Verification items for the finished model (mm, model axes). Coordinates: 2 decimals unless noted, no trailing zeros. Order: outer loops, then holes, each group sorted by start corner. A loop starts at its lowest first (then second) coordinate and runs counter-clockwise, first axis right, second up. Notation, with made-up numbers: (45, 36.25) -> (73, 36.25) arc R23 cw to (73, 75.25) -> close; hole circle Ø6 at (59.25, 60). An arc over 180 degrees is marked (long way). Answer as CSV lines item,"result".
```python
from build123d import *

# Parameters (mm, degrees)
SKETCH1_R           = 4
BOSS_EXTRUDE1_DEPTH = 6


with BuildPart() as part:
    # Sketch1 → Boss-Extrude1 (new body)
    with BuildSketch(Plane.XY):
        with BuildLine():
            Line((-80, 0), (-17.5, 0))
            ThreePointArc((-17.5, 0), (0, 17.5), (17.5, 0))
            Line((17.5, 0), (80, 0))
            ThreePointArc((80, 0), (0, 80), (-80, 0))
        make_face()
        with Locations((24.874423104, 60.052169613)):
            Circle(SKETCH1_R, mode=Mode.SUBTRACT)
        with Locations((60.052169613, 24.874423104)):
            Circle(SKETCH1_R, mode=Mode.SUBTRACT)
        with Locations((-60.052169613, 24.874423104)):
            Circle(SKETCH1_R, mode=Mode.SUBTRACT)
        with Locations(Location((-24.874423104, 60.052169613, 0), (0, 0, 180))):
            Circle(SKETCH1_R, mode=Mode.SUBTRACT)
    extrude(amount=BOSS_EXTRUDE1_DEPTH)


solid = part.part
```
Item 1: Section check B-B, the plane z = 3.6. Record the boundary of the cut face in (x, y).
Answer list:
outline,"(-80, 0) -> (-17.5, 0) arc R17.5 cw to (17.5, 0) -> (80, 0) arc R80 ccw to start; hole circle Ø8 at (-60.05, 24.87); hole circle Ø8 at (-24.87, 60.05); hole circle Ø8 at (24.87, 60.05); hole circle Ø8 at (60.05, 24.87)"
Item 2: Section check C-C, the plane x = 0. Record the boundary of the cut face in (y, z), plus the area to 3 significant figures.
Answer list:
outline,"(17.5, 0) -> (80, 0) -> (80, 6) -> (17.5, 6) -> close"
area,"375 mm2"
Item 3: Thickness scan on line 1 (X direction, y = 59.5, z = 5.7); line 2 (X direction, y = 5, z = 4.45); line 3 (X direction, y = 27, z = 1.6). Record the ranges inside material, lowest first.
Answer list:
line 1,"-53.48 to -28.84, -20.91 to 20.91, 28.84 to 53.48"
line 2,"-79.84 to -16.77, 16.77 to 79.84"
line 3,"-75.31 to -63.44, -56.66 to 56.66, 63.44 to 75.31"
Item 4: Depth check by flat-ended pin: pin 1 Ø4 at (x, y) = (28.5, 24) entering from -Z; pin 2 Ø7 at (x, y) = (-60.05, 24.87) entering from -Z; pin 3 Ø3 at (y, z) = (50.5, 1) entering from -X. Enter the tip coordinate at first touch or a pass-through.
Answer list:
pin 1,"z = 0"
pin 2,"through"
pin 3,"x = -63.24"
Item 5: Release check for a two-part mould opening along Y. For faces 1 (the cylindrical face through (-56.24, 26.08, 2.96)), 2 (the flat face through (-1, 41, 6)), 3 (the cylindrical face through (1.76, 79.98, 2.96)), 4 (the cylindrical face through (-24.007, 63.957, 2.958)) record: +Y half, -Y half, draft (parallel to the pull), parting line (faces both ways), or undercut.
Answer list:
face 1,"undercut"
face 2,"draft"
face 3,"+Y half"
face 4,"undercut"
Item 6: Section check D-D, the plane y = 31.5. Record the boundary of the cut face in (x, z), plus the area to 3 significant figures.
Answer list:
outline,"(-73.54, 0) -> (73.54, 0) -> (73.54, 6) -> (-73.54, 6) -> close"
area,"882 mm2"
Item 7: Section check A-A, the plane y = 7. Record the boundary of the cut face in (x, z).
Answer list:
outline,"(-79.69, 0) -> (-16.04, 0) -> (-16.04, 6) -> (-79.69, 6) -> close; (16.04, 0) -> (79.69, 0) -> (79.69, 6) -> (16.04, 6) -> close"
